from build123d import *

# Parameters (mm, degrees)
SKETCH2_R           = 4.3
BOSS_EXTRUDE2_DEPTH = 30
CUT_EXTRUDE2_DEPTH  = 18
SKETCH6_R           = 0.75
CUT_EXTRUDE3_DEPTH  = 10
SKETCH8_R           = 0.75
CUT_EXTRUDE5_DEPTH  = 5.3
SKETCH9_R           = 0.75
CUT_EXTRUDE6_DEPTH  = 10


with BuildPart() as part:
    # Sketch2 → Boss-Extrude2 (new body)
    with BuildSketch(Plane(origin=(0, 0, 0), x_dir=(1, 0, 0), z_dir=(0, 1, 0))):
        Circle(SKETCH2_R)
    extrude(amount=BOSS_EXTRUDE2_DEPTH)

    # Sketch4 → Cut-Extrude2 (cut)
    with BuildSketch(Plane(origin=(0, 30, 0), x_dir=(1, 0, 0), z_dir=(0, 1, 0))):
        with BuildLine():
            Line((0, 2.15), (-3.723909236, 2.15))
            ThreePointArc((-3.723909236, 2.15), (0, 4.3), (3.723909236, 2.15))
            Line((3.723909236, 2.15), (0, 2.15))
        make_face()
        with BuildLine():
            Line((0, -2.15), (-3.723909236, -2.15))
            ThreePointArc((-3.723909236, -2.15), (0, -4.3), (3.723909236, -2.15))
            Line((3.723909236, -2.15), (0, -2.15))
        make_face()
    extrude(amount=-CUT_EXTRUDE2_DEPTH, mode=Mode.SUBTRACT)

    # Sketch6 → Cut-Extrude3 (cut)
    with BuildSketch(Plane.XY.offset(2.15)):
        with Locations((0, 14)):
            Circle(SKETCH6_R)
    extrude(amount=-CUT_EXTRUDE3_DEPTH, mode=Mode.SUBTRACT)

    # Sketch8 → Cut-Extrude5 (cut, through all)
    with BuildSketch(Plane(origin=(0, 0, 0), x_dir=(0, 0, -1), z_dir=(1, 0, 0))):
        with Locations((0, 1)):
            Circle(SKETCH8_R)
    extrude(amount=-CUT_EXTRUDE5_DEPTH, mode=Mode.SUBTRACT)

    # Sketch9 → Cut-Extrude6 (cut)
    with BuildSketch(Plane.XY.offset(2.15)):
        with Locations((0, 28.5)):
            Circle(SKETCH9_R)
    extrude(amount=-CUT_EXTRUDE6_DEPTH, mode=Mode.SUBTRACT)


solid = part.part
The listing builds one solid part. Answer for the finished solid, in the listing's coordinates (mm). A direction names the side the tool comes from. Give positions to 0.01 mm unless a question says otherwise; leave off trailing zeros. Order: outer loops, then holes, each group sorted by start corner. A loop starts at its lowest first (then second) coordinate and runs counter-clockwise, first axis right, second up. Notation, with made-up numbers: (58.25, 82.5) - (66.25, 82.5) arc R9 cw to (66.25, 86.5) - close; hole circle Ø11 at (-2, -9.75). An arc over 180 degrees is marked (long way). One line per item, written item: value. Start each with the question number.
1) The mould has two halves that part along Z. Classify faces 4 (the face through (0, 12, 3)), 5 (the face through (-2.12, 0.268, 0.163)), 6 (the face through (3.97, 11.46, 1.65)): released by +Z, released by -Z, zero draft, split by the parting line, or undercut.
2) Find the intervals of material crossed by L1, parallel to Y at x = -1, z = 0; L2, parallel to Z at x = -3, y = 18.5, in increasing order.
3) A cutting plane is placed at B-B on z = 0. Give the vertices of the cut face in (x, y).
4) A cutting plane is placed at C-C on y = 8. Give the vertices of the cut face in (x, z), then the cut area to 3 significant figures.
5) A cutting plane is placed at A-A on y = 14. Give the vertices of the cut face in (x, z), then the cut area to 3 significant figures.
6) Given pin 1 Ø1.6 at (y, z) = (1, 0) entering from -X; pin 2 Ø4 at (x, y) = (2.5, 22.5) entering from +Z; pin 3 Ø0.9 at (x, y) = (0, 28.5) entering from -Z; pin 4 Ø3 at (x, y) = (3, 12.5) entering from +Z, each flat-ended and moving along its own axis, determine where each tip first touches the part or whether it passes through.
7) A cutting plane is placed at D-D on z = -3.25. Give the vertices of the cut face in (x, y).
8) A tool of negligible diameter and unlimited length cuts with its end or side. For faces 1 (the face through (0, 21, 2.15)), 2 (the face through (0, 21, -2.15)), 3 (the face through (0, 1, 0)), from which of +Z, -Z, +X, -X, +Y, -Y can it reach the whole face along a straight path? Write none if from no direction.
Answer sheet:
1. face 4: zero draft
1. face 5: undercut
1. face 6: split by the parting line
2. L1: y = 0 to 0.25, 1.75 to 30
2. L2: z = -2.15 to 2.15
3. outline: (-4.3, 0) - (4.3, 0) - (4.3, 30) - (-4.3, 30) - (-4.3, 1.75) - (0, 1.75) - (0, 0.25) - (-4.3, 0.25) - close; hole circle Ø1.5 at (0, 14); hole circle Ø1.5 at (0, 28.5)
4. outline: circle Ø8.6 at (0, 0)
4. area: 58.1 mm2
5. outline: (-3.72, -2.15) - (-0.75, -2.15) - (-0.75, 2.15) - (-3.72, 2.15) arc R4.3 ccw to start; (0.75, -2.15) - (3.72, -2.15) arc R4.3 ccw to (3.72, 2.15) - (0.75, 2.15) - close
5. area: 28.9 mm2
6. pin 1: stops at x = -4.3
6. pin 2: stops at z = 2.15
6. pin 3: passes through
6. pin 4: stops at z = 4
7. outline: (-2.82, 0) - (2.82, 0) - (2.82, 12) - (-2.82, 12) - close
8. face 1: +Z, +X, -X, +Y
8. face 2: -Z, +X, -X, +Y
8. face 3: -X
